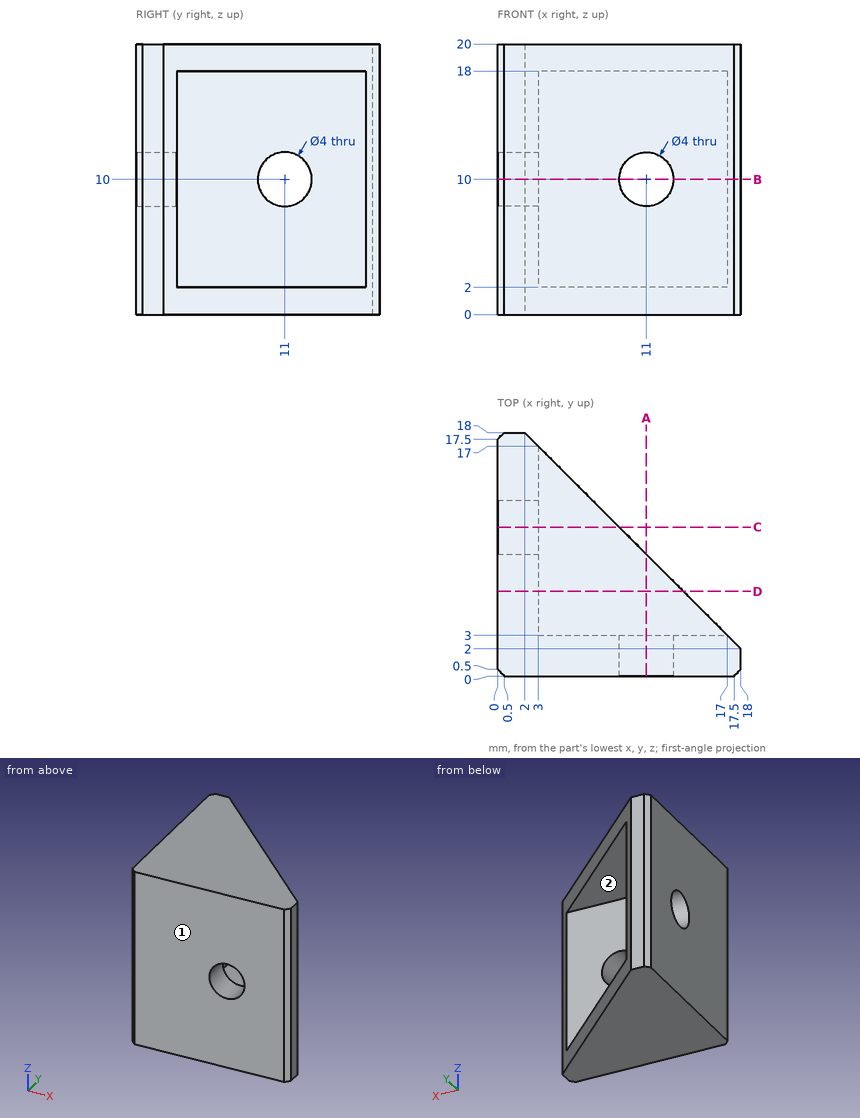
Geometry check sheet. Reference: drawing and pictorial views, mm from the part's lowest x, y, z. A direction names the side the tool comes from. Round coordinates to 2 decimals unless told otherwise and drop trailing zeros. Loops run counter-clockwise (first coordinate to the right, second up) from the corner with the lowest first, then second, coordinate; pieces in that order, holes last. Notation, with made-up numbers: M -35,-22.75 L -27,-22.75 A19 cw -27,5.25 Z; hole C -22.5,-18 d7. An arc over 180 degrees is marked long. One line per item, written item: value.
(1) Sectioned sample at B-B, the plane z = 10. Record the cut outline in (x, y), then the cut area to 3 significant figures.
Computed values:
outline: M 0,0.5 L 0.5,0 L 9,0 L 9,3 L 3,3 L 3,9 L 0,9 Z; M 0,13 L 3,13 L 3,17 L 2,18 L 0.5,18 L 0,17.5 Z; M 13,0 L 17.5,0 L 18,0.5 L 18,2 L 17,3 L 13,3 Z
area: 73.6 mm^2
(2) Access from +Z, -Z, +X, -X, +Y, -Y to the whole of each face (thin tool, end or side, straight path). Record for the marked faces 1 and 2.
Computed values:
face 1: +Z, -Z, +X, -X, -Y
face 2: +X, +Y
(3) Thickness scan on line 1 (X direction, y = 1.45, z = 10); line 2 (Z direction, x = 7.25, y = 11); line 3 (Z direction, x = 11, y = 2.1). Record the ranges inside material, lowest first.
Computed values:
line 1: x = 0 to 9, 13 to 18
line 2: z = 0 to 2, 18 to 20
line 3: z = 0 to 8, 12 to 20
(4) Sectioned sample at A-A, the plane x = 11. Record the cut outline in (y, z), then the cut area to 3 significant figures.
Computed values:
outline: M 0,0 L 9,0 L 9,2 L 3,2 L 3,8 L 0,8 Z; M 0,12 L 3,12 L 3,18 L 9,18 L 9,20 L 0,20 Z
area: 72.0 mm^2
(5) Sectioned sample at D-D, the plane y = 6.25. Record the cut outline in (x, z).
Computed values:
outline: M 0,0 L 13.75,0 L 13.75,2 L 3,2 L 3,18 L 13.75,18 L 13.75,20 L 0,20 Z
(6) Depth check by flat-ended pin: pin 1 Ø2 at (x, z) = (8.5, 17.5) entering from +Y; pin 2 Ø3.5 at (y, z) = (11, 10) entering from -X; pin 3 Ø4 at (x, z) = (10, 12.5) entering from +Y; pin 4 Ø1.5 at (x, z) = (13.5, 2.5) entering from +Y. Enter the tip coordinate at first touch or a pass-through.
Computed values:
pin 1: stops at y = 12.37
pin 2: passes through
pin 3: stops at y = 3
pin 4: stops at y = 7.06
